Source: CAD feature listing. Evaluate the final solid. Frame: model axes, mm. A direction names the side the tool comes from. Round coordinates to 2 decimals unless told otherwise and drop trailing zeros. Loops run counter-clockwise (first coordinate to the right, second up) from the corner with the lowest first, then second, coordinate; pieces in that order, holes last.
Item 1: Section query D-D on y = -72.5. Return loops of the section in (x, z), then the cut area to 3 significant figures.
Item 2: Ray query, L1, parallel to X at y = -672, z = 90.5; L2, parallel to Z at x = 52.5, y = -718. Return the intervals inside material, ascending.
Item 3: Section query C-C on z = 71. Return loops of the section in (x, y), then the cut area to 3 significant figures.
Item 4: Section query B-B on x = 11.5. Return loops of the section in (y, z).
Item 5: Pull-direction query (X, two-part tool) for faces 1 (the flat face through (49, -429, 100)), 2 (the flat face through (49, -426, 95)), 3 (the flat face through (100, -369, 49)); classes: released by +X, released by -X, zero draft, split by the parting line, or undercut.
Item 6: Section query A-A on y = -250.5. Return loops of the section in (x, z).
Item 7: First-contact query: P1, Ø5, axis at x = 69.5, y = -92.5, coming from the +Z side. Flat tip, straight axial feed; report the tip coordinate or a pass-through.
Item 8: Access query for faces 4 (the flat face through (0, -369, 49)), 5 (the flat face through (5, -372, 49)). Directions: +Z, -Z, +X, -X, +Y, -Y. A direction counts if a zero-diameter tool reaches every point of the face in a straight line with its end or side. Return the directions, or none.
```python
from build123d import *

# Parameters (mm, degrees)
F0_W     = 100
F0_H     = 100
F0_W_2   = 90
F0_H_2   = 90
F1_DEPTH = 750
F3_DEPTH = 100.001
F5_DEPTH = 100.001


with BuildPart() as f1:
    # F0 (on Front) → F1 (new body)
    with BuildSketch(Plane.XZ):
        with Locations((50, 50)):
            Rectangle(F0_W, F0_H)
        with Locations((50, 50)):
            Rectangle(F0_W_2, F0_H_2, mode=Mode.SUBTRACT)
    extrude(amount=F1_DEPTH)

    # F2 (on face) → F3 (cut, through all)
    with BuildSketch(Plane.YZ.offset(100)):
        Polygon((-679.944465, 120), (-755, 120), (-755, -10), align=None)
    extrude(amount=-F3_DEPTH, mode=Mode.SUBTRACT)

    # F4 (on face) → F5 (cut, through all)
    with BuildSketch(Plane.YZ.offset(100)):
        Polygon((0.141252, 114.146464), (-197.538123, 114.146464), (0.141252, 0.016223), align=None)
    extrude(amount=-F5_DEPTH, mode=Mode.SUBTRACT)


solid = f1.part
```
Data:
1. outline: (0, 0) - (100, 0) - (100, 41.96) - (95, 41.96) - (95, 5) - (5, 5) - (5, 41.96) - (0, 41.96) - close
1. area: 870 mm2
2. L1: x = 0 to 5, 95 to 100
2. L2: z = 0 to 5
3. outline: (0, -708.23) - (5, -708.23) - (5, -122.81) - (0, -122.81) - close; (95, -708.23) - (100, -708.23) - (100, -122.81) - (95, -122.81) - close
3. area: 5,850 mm2
4. outline: (-749.23, 0) - (0, 0) - (0, 0.1) - (-8.49, 5) - (-746.34, 5) - close; (-694.38, 95) - (-164.38, 95) - (-173.04, 100) - (-691.49, 100) - close
5. face 1: zero draft
5. face 2: undercut
5. face 3: released by +X
6. outline: (0, 0) - (100, 0) - (100, 100) - (0, 100) - close; hole (5, 5) - (95, 5) - (95, 95) - (5, 95) - close
7. P1: stops at z = 5
8. face 4: +Z, -Z, -X, +Y, -Y
8. face 5: +Y, -Y
